from build123d import *

# Parameters (mm, degrees)
F1_DEPTH = 15
F2_R     = 4.99999
F3_R     = 2


# Not quite as in the source:
# - a fillet or chamfer is up to 0.001 mm smaller than in the source, because OpenCascade refuses the exact size


with BuildPart() as f1:
    # F0 (on Top) → F1 (new body)
    with BuildSketch(Plane.XY):
        Polygon((0, 10), (0, 0), (42.567110899, 0), (88.8907263303, 127.2730873849), (79.4938001224, 130.6932888181), (35.5650355169, 10), align=None)
    extrude(amount=F1_DEPTH)

    # F2 (radius 5 in the source; OpenCascade refuses exactly that, so slightly less here)
    f2_edges = [f1.edges().sort_by_distance(p)[0] for p in [
        (35.565036, 10, 7.5),
        (42.567111, 0, 7.5),
        (79.4938, 130.693289, 7.5),
        (88.890726, 127.273087, 7.5),
    ]]
    fillet(f2_edges, radius=F2_R)

    # F3
    f3_edges = [f1.edges().sort_by_distance(p)[0] for p in [
        (57.273081, 69.642364, 15),
        (57.273081, 69.642364, 0),
    ]]
    fillet(f3_edges, radius=F3_R)


solid = f1.part
For this review, take the finished solid that the model builds, in its own axes (mm). A direction names the side the tool comes from. Round coordinates to 2 decimals unless told otherwise and drop trailing zeros. Write each loop counter-clockwise with the first axis right and the second up, starting at its lowest first coordinate (ties: lowest second). Pieces come first, ordered by that corner, then holes. Notation, with made-up numbers: (47, 50.25) - (80, 50.25) arc R34 cw to (80, 84.25) - close; hole circle Ø4 at (-23, 9.5). An arc over 180 degrees is marked (long way). Write item = value, one per line. Start each with the question number.
1. For pin 1 Ø4 at (y, z) = (70.5, 4.5) entering from -X; pin 2 Ø3.5 at (x, z) = (19, 5) entering from +Y; pin 3 Ø5 at (x, z) = (42.5, 7) entering from -Y, all flat-tipped, find the tip position at first contact; note any pin that passes through.
2. For faces 1 (the face through (65.21, 63.97, 14.43)), 2 (the face through (16, 10, 7)), list the 3-axis set-ups (+Z, -Z, +X, -X, +Y, -Y) from which the entire face can be reached by the end or side of a thin tool; tool diameter is ignored.
3. Wall thickness on L1, parallel to Y at x = 26, z = 12.5; L2, parallel to X at y = 9, z = 6.5; L3, parallel to X at y = 108, z = 14: over which ranges is each line inside the solid? List them lowest first.
4. Draft analysis for pull direction X (two halves, no side actions). For faces 3 (the face through (80.42, 128.84, 7.58)), 4 (the face through (0, 5, 7)), 5 (the face through (65.17, 62.1, 7.42)), 6 (the face through (19, 0, 7)), state which applies: released by +X, released by -X, zero draft, split by the parting line, or undercut.
5. Consider section A-A on x = 6. State the section outline as (y, z) points, plus the area to 3 significant figures.
Evaluation:
q1.pin_1 = 56.86
q1.pin_2 = 10
q1.pin_3 = 0.09
q2.face_1 = +Z, +X, -Y
q2.face_2 = +Z, -Z, -X, +Y
q3.L1 = 0 to 10
q3.L2 = 0 to 45.84
q3.L3 = 71.52 to 81.59
q4.face_3 = split by the parting line
q4.face_4 = released by -X
q4.face_5 = released by +X
q4.face_6 = zero draft
q5.outline = (0, 2) arc R2 ccw to (2, 0) - (8, 0) arc R2 ccw to (10, 2) - (10, 13) arc R2 ccw to (8, 15) - (2, 15) arc R2 ccw to (0, 13) - close
q5.area = 147 mm2
